Read the model definition and answer for the solid it produces. Units are mm, in the model's axes. A direction names the side the tool comes from. Coordinates: 2 decimals unless noted, no trailing zeros. Loops run counter-clockwise (first coordinate to the right, second up) from the corner with the lowest first, then second, coordinate; pieces in that order, holes last. Notation, with made-up numbers: (75, 86) -> (88, 86) arc R21 cw to (88, 125) -> close; hole circle Ø10 at (27, 85.25). An arc over 180 degrees is marked (long way). Answer as a JSON object with one key per item and string values. Group by question number.
Q1. For faces 1 (the flat face through (-35.75, 0, 21)), 2 (the flat face through (1, 19.75, 21)), 3 (the flat face through (1, -19.75, 21)), 4 (the flat face through (38.5, 0, 37)), 5 (the flat face through (-37, -7.5, 33)), determine the directions among +Z, -Z, +X, -X, +Y, -Y from which every point of the face is accessible in a straight line to the end or side of a thin tool.
Q2. The part is cut by section C-C on z = 33.5. Write down the section's boundary in (x, y).
Q3. The part is cut by section B-B on y = 16. Write down the section's boundary in (x, z), and give its area (3 significant figures).
Q4. Straight lines are drawn through the part: line 1 along Y through (x, z) = (10, 12); line 2 along X through (y, z) = (1.5, 20); line 3 along X through (y, z) = (0, 38.5). For each, find the intervals that lie inside material, in ascending order. Write a range as [from, to].
Q5. Each of these flat-tipped pins is pushed along its axis until it touches: P1, Ø8, axis at y = -17, z = 14, coming from the +X side; P2, Ø3, axis at x = -37, z = 35, coming from the -Y side; P3, Ø1.4, axis at x = 37, z = 29, coming from the +Y side. Where does it stop, or does it pass through?
Q6. The part is cut by section A-A on x = 22. Write down the section's boundary in (y, z).
Q7. The part is cut by section D-D on y = -3.5. Write down the section's boundary in (x, z), and give its area (3 significant figures).
from build123d import *

# Parameters (mm, degrees)
SKIZZE1_W                       = 79
SKIZZE1_H                       = 43
AUFSATZ_LINEAR_AUSTRAGEN1_DEPTH = 45
SKIZZE2_W                       = 79
SKIZZE2_H                       = 43
SKIZZE2_W_2                     = 71.5
SKIZZE2_H_2                     = 39.5
SCHNITT_LINEAR_AUSTRAGEN1_DEPTH = 43
SKIZZE3_W                       = 2.75
SKIZZE3_H                       = 15
AUFSATZ_LINEAR_AUSTRAGEN2_DEPTH = 20
VERRUNDUNG1_R                   = 10


with BuildPart() as part:
    # Skizze1 → Aufsatz-Linear austragen1 (new body)
    with BuildSketch(Plane.XY):
        Rectangle(SKIZZE1_W, SKIZZE1_H)
    extrude(amount=AUFSATZ_LINEAR_AUSTRAGEN1_DEPTH)

    # Skizze2 → Schnitt-Linear austragen1 (cut)
    with BuildSketch(Plane(origin=(0, 0, 0), x_dir=(-1, 0, 0), z_dir=(0, 0, -1))):
        Rectangle(SKIZZE2_W, SKIZZE2_H)
        Rectangle(SKIZZE2_W_2, SKIZZE2_H_2, mode=Mode.SUBTRACT)
    extrude(amount=-SCHNITT_LINEAR_AUSTRAGEN1_DEPTH, mode=Mode.SUBTRACT)

    # Skizze3 → Aufsatz-Linear austragen2 (add)
    with BuildSketch(Plane(origin=(0, 0, 43), x_dir=(-1, 0, 0), z_dir=(0, 0, -1))):
        with Locations((-37.125, 0)):
            Rectangle(SKIZZE3_W, SKIZZE3_H)
        with Locations((37.125, 0)):
            Rectangle(SKIZZE3_W, SKIZZE3_H)
    extrude(amount=AUFSATZ_LINEAR_AUSTRAGEN2_DEPTH)

    # Verrundung1
    # the kernel refuses this fillet: 10 mm, written as the material it takes off along each edge
    with BuildSketch(Plane(origin=(-38.5, 24.718721642, 23), x_dir=(0, 0, 1), z_dir=(0, -1, 0)), Plane(origin=(38.5, -24.718721642, 23), x_dir=(0, 0, 1), z_dir=(0, 1, 0))) as verrundung1_piece_1:
        with BuildLine():
            CenterArc((6.887488657, -10), VERRUNDUNG1_R, 90, 43.531152167)
            Line((0, -2.75), (-0.137749773, -2.605))
            ThreePointArc((-0.137749773, -2.605), (-0.2, -1.375), (-0.2, 0))
            Line((-0.2, 0), (0, 0.2))
            Line((0, 0.2), (6.887488657, 0.2))
            Line((6.887488657, 0.2), (6.887488657, 0))
        make_face()
    extrude(amount=49.437443285, mode=Mode.SUBTRACT)


solid = part.part
Final values:
{
 "1": {"face 1": "-Z, -X", "face 2": "-Z, +X, -X, +Y", "face 3": "-Z, +X, -X, -Y", "face 4": "-Z, +X, +Y, -Y", "face 5": "-Z, -X, -Y"},
 "2": {"outline": "(-38.5, -7.5) -> (-35.75, -7.5) -> (-35.75, -19.75) -> (35.75, -19.75) -> (35.75, -7.5) -> (38.5, -7.5) -> (38.5, 7.5) -> (35.75, 7.5) -> (35.75, 19.75) -> (-35.75, 19.75) -> (-35.75, 7.5) -> (-38.5, 7.5) -> close"},
 "3": {"outline": "(-39.5, 43) -> (-35.75, 43) -> (-35.75, 0) -> (35.75, 0) -> (35.75, 43) -> (39.5, 43) -> (39.5, 45) -> (-39.5, 45) -> close", "area": "3,230 mm2"},
 "4": {"line 1": "y = [-19.75, 19.75]", "line 2": "x = [-35.75, 35.75]", "line 3": "x = [-38.5, 38.5]"},
 "5": {"P1": "stops at x = 35.75", "P2": "stops at y = -19.75", "P3": "stops at y = 7.5"},
 "6": {"outline": "(-21.5, 43) -> (-19.75, 43) -> (-19.75, 0) -> (19.75, 0) -> (19.75, 43) -> (21.5, 43) -> (21.5, 45) -> (-21.5, 45) -> close"},
 "7": {"outline": "(-39.5, 43) -> (-38.5, 43) -> (-38.5, 29.89) arc R10 ccw to (-35.75, 23) -> (-35.75, 0) -> (35.75, 0) -> (35.75, 23) arc R10 ccw to (38.5, 29.89) -> (38.5, 43) -> (39.5, 43) -> (39.5, 45) -> (-39.5, 45) -> close", "area": "3,330 mm2"}
}
